```python
from build123d import *

# Parameters (mm, degrees)
F1_W           = 50.8
F1_H           = 19.05
F2_DEPTH       = 2.3876
F2_DEPTH_BACK  = 2.3876
F3_R           = 5.08
F4_R           = 6.35
F5_R           = 6.35
F7_D           = 11.1125
F9_D           = 11.1125
F11_D          = 6.35
F13_DEPTH      = 2.3876
F13_DEPTH_BACK = 2.3876
F15_DEPTH      = 2.3876
F15_DEPTH_BACK = 2.3876
F16_T1_DEPTH   = 4.7752
F16_T6_DEPTH   = 4.7752
F17_R          = 0.508


# Not quite as in the source:
# - a fillet or chamfer that OpenCascade refuses, or shapes differently, is made with other operations: its cross-section is extruded or revolved along the edge and cut away or added


with BuildPart() as f2:
    # F1 (on face) → F2 (new body, two sides)
    with BuildSketch(Plane.XZ) as f2_sk:
        with Locations((-6.4059151608, 1.9555166364)):
            Rectangle(F1_W, F1_H)
    extrude(amount=F2_DEPTH)
    extrude(f2_sk.sketch, amount=-F2_DEPTH_BACK)

    # F3
    f3_edges = [f2.edges().sort_by_distance(p)[0] for p in [
        (18.994085, 0, 11.480517),
    ]]
    fillet(f3_edges, radius=F3_R)

    # F4
    f4_edges = [f2.edges().sort_by_distance(p)[0] for p in [
        (18.994085, 0, -7.569483),
    ]]
    fillet(f4_edges, radius=F4_R)

    # F5
    f5_edges = [f2.edges().sort_by_distance(p)[0] for p in [
        (-31.805915, 0, 11.480517),
        (-31.805915, 0, -7.569483),
    ]]
    fillet(f5_edges, radius=F5_R)

    # F7 (through all)
    with Locations(Plane.XZ.offset(2.3876)):
        with Locations((9.4690848392, 1.9555166364)):
            Hole(F7_D / 2)

    # F9 (through all)
    with Locations(Plane.XZ.offset(2.3876)):
        with Locations((-22.2809151608, 1.9555166364)):
            Hole(F9_D / 2)

    # F11 (through all)
    with Locations(Plane.XZ.offset(2.3876)):
        with Locations((-6.4059151608, 1.9555166364)):
            Hole(F11_D / 2)

    # F12 (on Front) → F13 (join, two sides)
    with BuildSketch(Plane.XZ) as f13_sk:
        Polygon((8.6054187268, 40.0424157364), (4.6366687268, 40.0424157364), (4.6366687268, 11.4674157364), (12.5741687268, 11.4674157364), (12.5741687268, 40.0424157364), align=None)
    extrude(amount=F13_DEPTH)
    extrude(f13_sk.sketch, amount=-F13_DEPTH_BACK)

    # F14 (on Front) → F15 (join, two sides)
    with BuildSketch(Plane.XZ) as f15_sk:
        with BuildLine():
            Line((18.1304187268, 40.0424157364), (8.6054187268, 71.7924157364))
            ThreePointArc((8.6054187268, 71.7924157364), (1.180386736, 56.7161753336), (-0.9195812732, 40.0424157364))
            Line((-0.9195812732, 40.0424157364), (8.6054187268, 40.0424157364))
            Line((8.6054187268, 40.0424157364), (18.1304187268, 40.0424157364))
        make_face()
    extrude(amount=F15_DEPTH)
    extrude(f15_sk.sketch, amount=-F15_DEPTH_BACK)

    # F16: fillet of radius 6.35 on 2 edges, made by hand

    # F16_s2 → F16_t1 (join)
    with BuildSketch(Plane.XZ.offset(-2.3876)):
        with BuildLine():
            ThreePointArc((-0.9195812732, 40.0424157364), (3.0491687268, 37.9423506332), (4.6366687268, 33.7422204269))
            Line((4.6366687268, 33.7422204269), (4.7636687268, 33.7422204269))
            Line((4.7636687268, 33.7422204269), (4.7636687268, 40.0424157364))
            Line((4.7636687268, 40.0424157364), (4.6366687268, 40.1694157364))
            ThreePointArc((4.6366687268, 40.1694157364), (1.8585437268, 40.1694157364), (-0.9037062732, 40.1684196426))
            Line((-0.9037062732, 40.1684196426), (-0.9195812732, 40.0424157364))
        make_face()
    extrude(amount=F16_T1_DEPTH)


with BuildPart() as f16_tool4:
    # F16_s5 → F16_t6 (new body)
    with BuildSketch(Plane.XZ.offset(2.3876)):
        with BuildLine():
            ThreePointArc((18.1304187268, 40.0424157364), (14.1616687268, 37.9423506332), (12.5741687268, 33.7422204269))
            Line((12.5741687268, 33.7422204269), (12.4471687268, 33.7422204269))
            Line((12.4471687268, 33.7422204269), (12.4471687268, 40.0424157364))
            Line((12.4471687268, 40.0424157364), (12.5741687268, 40.1694157364))
            ThreePointArc((12.5741687268, 40.1694157364), (15.3522937268, 40.1694157364), (18.1145437268, 40.1684196426))
            Line((18.1145437268, 40.1684196426), (18.1304187268, 40.0424157364))
        make_face()
    extrude(amount=-F16_T6_DEPTH)

    split(bisect_by=Plane(origin=(27.6542600438, 0, 8.2962780131), x_dir=(0, 1, 0), z_dir=(-0.9578262852, 0, -0.2873478856)), keep=Keep.TOP)


with BuildPart() as f2_1:
    add(f2.part)

    # F16_t3: union F16_tool4
    add(f16_tool4.part)

    # F17
    f17_edges = [f2_1.edges().sort_by_distance(p)[0] for p in [
        (18.130419, 0, 40.042416),
        (-0.919581, 0, 40.042416),
    ]]
    fillet(f17_edges, radius=F17_R)


solid = f2_1.part
```
Read the model definition and answer for the solid it produces. Units are mm, in the model's axes. A direction names the side the tool comes from. Give positions to 0.01 mm unless a question says otherwise; leave off trailing zeros. Order: outer loops, then holes, each group sorted by start corner. A loop starts at its lowest first (then second) coordinate and runs counter-clockwise, first axis right, second up.
(1) Find section D-D (y = 1.25). Give the number of separate pieces and of enclosed holes in the cut face, plus the area to 3 significant figures.
(2) Straight lines are drawn through the part: L1, parallel to Z at x = -6.5, y = -0.3; L2, parallel to X at y = -0.35, z = -1.5; L3, parallel to X at y = -0.8, z = 6.5. For each, find the intervals that lie inside material, in ascending order.
(3) Find section C-C (x = 6). Give the vertices of the cut face in (y, z), plus the area to 3 significant figures.
(4) Find section B-B (z = 20). Give the vertices of the cut face in (x, y).
(5) For faces 4 (the flat face through (12.574, 0, 22)), 5 (the flat face through (-11, 0, 11.481)), 6 (the flat face through (5, 2.388, 18)), determine the directions among +Z, -Z, +X, -X, +Y, -Y from which every point of the face is accessible in a straight line to the end or side of a thin tool.
(6) Given pin 1 (1 mm diameter, centred on x = -11.5, y = -0.5, fed in from +Z); pin 2 (6.5 mm diameter, centred on x = 9.47, z = 1.96, fed in from +Y), each flat-ended and moving along its own axis, determine where each tip first touches the part or whether it passes through.
(7) For a pull along Z with two mould halves and no side action, classify faces 1 (the cylindrical face through (17.183, -0.033, -5.66)), 2 (the cylindrical face through (-3.234, 0.033, 2.095)), 3 (the flat face through (-31.806, 0, 2)) as released by +Z, released by -Z, zero draft, split by the parting line, or undercut.
(8) Find section A-A (x = -17.5). Give the vertices of the cut face in (y, z).
Result sheet:
1. separate pieces: 1
1. enclosed holes: 3
1. area: 1,320 mm2
2. L1: z = -7.57 to -1.22, 5.13 to 11.48
2. L2: x = -31.8 to -26.63, -17.93 to 5.12, 13.82 to 18.99
2. L3: x = -31.66 to -25.48, -19.08 to 6.27, 12.67 to 18.99
3. outline: (-2.39, -7.57) - (2.39, -7.57) - (2.39, -2.38) - (-2.39, -2.38) - close; (-2.39, 6.3) - (2.39, 6.3) - (2.39, 67.79) - (-2.39, 67.79) - close
3. area: 318 mm2
4. outline: (4.64, -2.39) - (12.57, -2.39) - (12.57, 2.39) - (4.64, 2.39) - close
5. face 4: +X, +Y, -Y
5. face 5: -X, +Y, -Y
5. face 6: +Z, -Z, +X, -X, +Y
6. pin 1: stops at z = 11.48
6. pin 2: passes through
7. face 1: released by -Z
7. face 2: undercut
7. face 3: zero draft
8. outline: (-2.39, -7.57) - (2.39, -7.57) - (2.39, -0.88) - (-2.39, -0.88) - close; (-2.39, 4.79) - (2.39, 4.79) - (2.39, 11.48) - (-2.39, 11.48) - close
